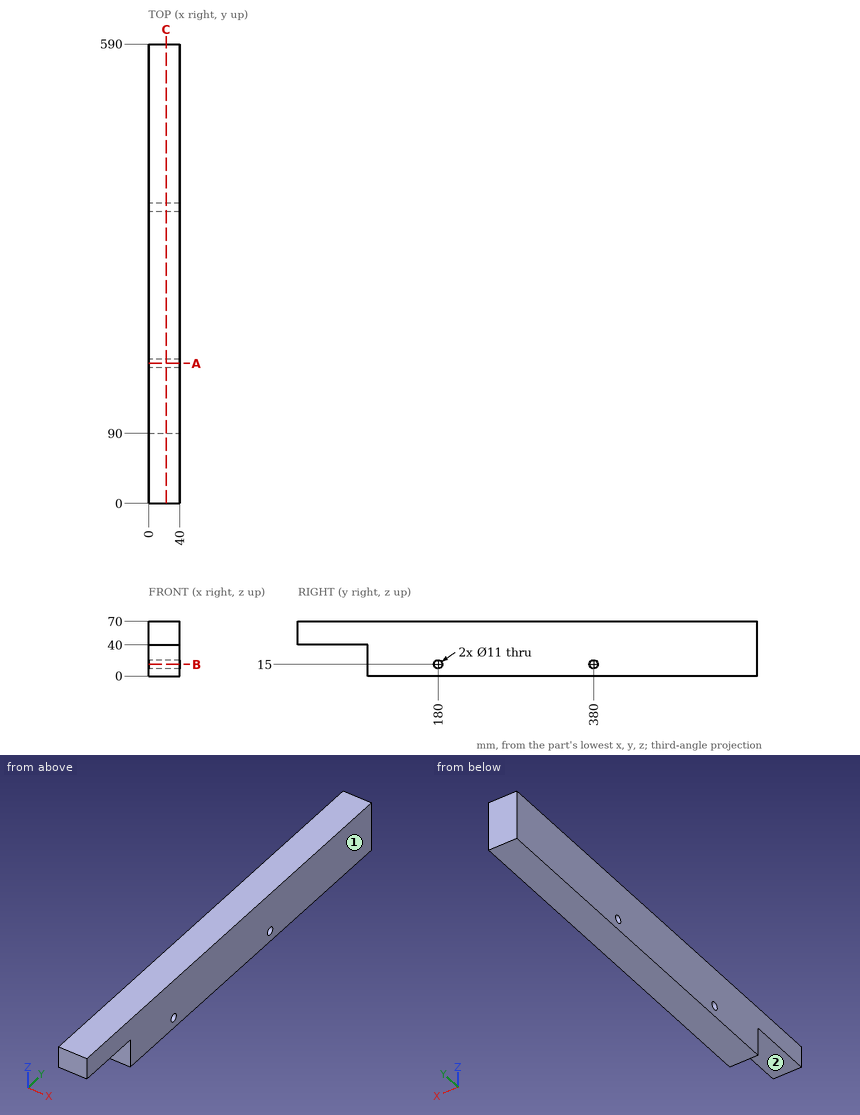
Job drawing, mm, ordinate dimensions from the low corner. One solid piece. A direction names the side the tool comes from. Give positions to 0.01 mm unless a question says otherwise; leave off trailing zeros. Write each loop counter-clockwise with the first axis right and the second up, starting at its lowest first coordinate (ties: lowest second). Pieces come first, ordered by that corner, then holes. Notation, with made-up numbers: (88.25, 74) -> (145.25, 74) arc R25 ccw to (145.25, 107) -> close; hole circle Ø11 at (20, 29.5). An arc over 180 degrees is marked (long way). Return JSON: item names as keys, results as strings.
Item 1: Band-saw the part on A-A (y = 180). List the corners of the cut face in (x, z), then the cut area to 3 significant figures.
Answer below:
{"outline": "(0, 0) -> (40, 0) -> (40, 9.5) -> (0, 9.5) -> close; (0, 20.5) -> (40, 20.5) -> (40, 70) -> (0, 70) -> close", "area": "2,360 mm2"}
Item 2: Band-saw the part on C-C (x = 22.5). List the corners of the cut face in (y, z).
Answer below:
{"outline": "(0, 40) -> (90, 40) -> (90, 0) -> (590, 0) -> (590, 70) -> (0, 70) -> close; hole circle Ø11 at (180, 15); hole circle Ø11 at (380, 15)"}
Item 3: Drop flat-ended pins along their axis: pin 1 (12 mm diameter, centred on x = 29.5, y = 62.5, fed in from -Z); pin 2 (10 mm diameter, centred on y = 380, z = 15, fed in from -X); pin 3 (1 mm diameter, centred on x = 16.5, z = 16.5, fed in from -Y). Give the stop position or say it passes through.
Answer below:
{"pin 1": "stops at z = 40", "pin 2": "passes through", "pin 3": "stops at y = 90"}
Item 4: Tool access for the marked faces 1 and 2: list every direction of +Z, -Z, +X, -X, +Y, -Y with a clear straight run to the whole face (end or side of a thin tool).
Answer below:
{"face 1": "+Z, -Z, +X, +Y, -Y", "face 2": "-Z, +X, -X, -Y"}
Item 5: Band-saw the part on B-B (z = 15). List the corners of the cut face in (x, y), then the cut area to 3 significant figures.
Answer below:
{"outline": "(0, 90) -> (40, 90) -> (40, 174.5) -> (0, 174.5) -> close; (0, 185.5) -> (40, 185.5) -> (40, 374.5) -> (0, 374.5) -> close; (0, 385.5) -> (40, 385.5) -> (40, 590) -> (0, 590) -> close", "area": "19,100 mm2"}
Item 6: Drill centre lines: probe 1 along Y at (x, z) = (23.5, 14); probe 2 along Z at (x, y) = (12, 180); probe 3 along Y at (x, z) = (7, 10.5). Where is each one in solid material? Low to high.
Answer below:
{"probe 1": "y = 90 to 174.59, 185.41 to 374.59, 385.41 to 590", "probe 2": "z = 0 to 9.5, 20.5 to 70", "probe 3": "y = 90 to 176.84, 183.16 to 376.84, 383.16 to 590"}
